Autodesk Inventor part; units mm, degrees
ref_plane "YZ Plane" through (0, 0, 0) normal (1, 0, 0) x (0, 1, 0)
ref_plane "XZ Plane" through (0, 0, 0) normal (0, 1, 0) x (-1, 0, 0)
ref_plane "XY Plane" through (0, 0, 0) normal (0, 0, 1) x (1, 0, 0)
sketch "Sketch1" plane through (0, 0, 0) normal (0, 0, 1) x (1, 0, 0)
  line L0 (0, 0) -> (110, 0)
  line L1 (110, 0) -> (110, 60)
  line L2 (110, 60) -> (0, 60)
  line L3 (0, 60) -> (0, 0)
  dimension "d0" = 60
  dimension "d1" = 110
extrude "Extrusion1" add sketch "Sketch1" along normal blind 3
sketch "Sketch2" plane through (0, 0, 3) normal (0, 0, 1) x (1, 0, 0)
  line L0 (0, 0) -> (110, 0)
  line L1 (0, 0) -> (10, 0)
  line L2 (10, 0) -> (10, -3)
  line L3 (10, -3) -> (0, -3)
  line L4 (0, -3) -> (0, 0)
  line L5 (20, 0) -> (30, 0)
  line L6 (30, 0) -> (30, -3)
  line L7 (30, -3) -> (20, -3)
  line L8 (20, -3) -> (20, 0)
  line L9 (40, 0) -> (50, 0)
  line L10 (50, 0) -> (50, -3)
  line L11 (50, -3) -> (40, -3)
  line L12 (40, -3) -> (40, 0)
  line L13 (60, 0) -> (70, 0)
  line L14 (70, 0) -> (70, -3)
  line L15 (70, -3) -> (60, -3)
  line L16 (60, -3) -> (60, 0)
  line L17 (80, 0) -> (90, 0)
  line L18 (90, 0) -> (90, -3)
  line L19 (90, -3) -> (80, -3)
  line L20 (80, -3) -> (80, 0)
  line L21 (100, 0) -> (110, 0)
  line L22 (110, 0) -> (110, -3)
  line L23 (110, -3) -> (100, -3)
  line L24 (100, -3) -> (100, 0)
  line L25 (0, 60) -> (0, 0) construction
  dimension "d4" = 10
  dimension "d5" = 3
  dimension "d8" = 20
extrude "Extrusion2" add sketch "Sketch2" against normal blind 3
sketch "Sketch3" plane through (0, 0, 3) normal (0, 0, 1) x (1, 0, 0)
  line L0 (-3, 20) -> (0, 20)
  line L1 (0, 20) -> (0, 10)
  line L2 (0, 10) -> (-3, 10)
  line L3 (-3, 10) -> (-3, 20)
  line L4 (0, 63) -> (0, -3) construction
  line L5 (10, 0) -> (20, 0) construction
  line L6 (-3, 40) -> (0, 40)
  line L7 (0, 40) -> (0, 30)
  line L8 (0, 30) -> (-3, 30)
  line L9 (-3, 30) -> (-3, 40)
  line L10 (-3, 60) -> (0, 60)
  line L11 (0, 60) -> (0, 50)
  line L12 (0, 50) -> (-3, 50)
  line L13 (-3, 50) -> (-3, 60)
  line L14 (110, 20) -> (113, 20)
  line L15 (113, 20) -> (113, 10)
  line L16 (113, 10) -> (110, 10)
  line L17 (110, 10) -> (110, 20)
  line L18 (110, 40) -> (113, 40)
  line L19 (113, 40) -> (113, 30)
  line L20 (113, 30) -> (110, 30)
  line L21 (110, 30) -> (110, 40)
  line L22 (110, 60) -> (113, 60)
  line L23 (113, 60) -> (113, 50)
  line L24 (113, 50) -> (110, 50)
  line L25 (110, 50) -> (110, 60)
  point P0 (0, 0)
  dimension "d16" = 3
  dimension "d17" = 10
  dimension "d18" = 10
  dimension "d21" = 20
  dimension "d24" = 113
extrude "Extrusion3" add sketch "Sketch3" against normal blind 3
properties part number "portada"
The model under review builds one solid part; all positions refer to its coordinate system, in mm. A direction names the side the tool comes from. Round coordinates to 2 decimals unless told otherwise and drop trailing zeros. Write each loop counter-clockwise with the first axis right and the second up, starting at its lowest first coordinate (ties: lowest second). Pieces come first, ordered by that corner, then holes.
(1) Machinability: for faces 5 (the flat face through (110, 3, 1)), 6 (the flat face through (110, 25, 1)), 7 (the flat face through (0, 25, 1)), 8 (the flat face through (40, -2, 2)), which of the approach directions +Z, -Z, +X, -X, +Y, -Y give a long, thin tool a straight path to every point of the face, cutting with its end or side? Answer none if there is none.
(2) Insertion check: pin 1 (0.9 mm diameter, centred on y = -1, z = 1, fed in from +X); pin 2 (1.5 mm diameter, centred on y = -2, z = 1.5, fed in from -X); pin 3 (1.5 mm diameter, centred on x = 94, z = 1.5, fed in from -Y). Each pin has a flat end and moves straight along its axis. Give the tip position at first contact, or say it passes through.
(3) Wall thickness on L1, parallel to X at y = 28.5, z = 2.7; L2, parallel to Y at x = 35, z = 2.45: over which ranges is each line inside the solid? List them lowest first.
(4) We need section B-B on x = 17. Give the boundary of the cut face in (y, z), and give its area (3 significant figures).
(5) Mouldability with a two-part tool opening along Y and no side actions: class faces 1 (the flat face through (113, 55, 2)), 2 (the flat face through (15, 0, 1)), 3 (the flat face through (112, 30, 2)), 4 (the flat face through (-2, 20, 2)) as +Y half, -Y half, draft (parallel to the pull), parting line (faces both ways), or undercut.
(6) We need section A-A on y = 5.5. Give the boundary of the cut face in (x, z).
Findings below:
1. face 5: +Z, -Z, +X, -Y
1. face 6: +Z, -Z, +X
1. face 7: +Z, -Z, -X
1. face 8: +Z, -Z, -Y
2. pin 1: stops at x = 110
2. pin 2: stops at x = 0
2. pin 3: stops at y = 0
3. L1: x = 0 to 110
3. L2: y = 0 to 60
4. outline: (0, 0) - (60, 0) - (60, 3) - (0, 3) - close
4. area: 180 mm2
5. face 1: draft
5. face 2: -Y half
5. face 3: undercut
5. face 4: undercut
6. outline: (0, 0) - (110, 0) - (110, 3) - (0, 3) - close
